Here's how the part is built. I have some questions about the finished solid (model axes, mm). A direction names the side the tool comes from. Give positions to 0.01 mm unless a question says otherwise; leave off trailing zeros. Write each loop counter-clockwise with the first axis right and the second up, starting at its lowest first coordinate (ties: lowest second). Pieces come first, ordered by that corner, then holes. Notation, with made-up numbers: (17.25, 49) - (76.25, 49) arc R16 cw to (76.25, 57) - close; hole circle Ø5 at (28, 18). An arc over 180 degrees is marked (long way). Write each question's results on one line, items separated by ' | '. Start each with the question number.
Item 1: We'd pull the mould along X, two halves only. Please class faces 6 (the cylindrical face through (-23.43, 4.93, 83.45)), 7 (the cylindrical face through (0.22, 6.084, -30.907)), 8 (the cylindrical face through (-65.4, 12.5, 43.2)): +X half, -X half, draft (parallel to the pull), parting line (faces both ways), or undercut.
Item 2: Suppose I cut it at C-C on z = 79. List the corners of the cut face in (x, y) for me.
Item 3: Will these pins go through, and if not, where does the flat tip stop? P1, Ø17.5, axis at x = -54, z = -25.5, coming from the -Y side; P2, Ø1.5, axis at x = 12.5, z = -63.5, coming from the -Y side; P3, Ø4, axis at x = 8.5, y = 13, coming from the -Z side.
Item 4: Which directions (+Z, -Z, +X, -X, +Y, -Y) give clear straight access to the entire face, cutting with the end or side of a thin tool? Please do faces 1 (the cylindrical face through (-65.67, 12.54, 16.84)), 2 (the cylindrical face through (1.033, 12.535, 54.773)), 3 (the flat face through (63.557, 12, -26)), 4 (the cylindrical face through (-59.669, 8.986, -12.754)), 5 (the cylindrical face through (46.448, 12.535, -93.326)).
Item 5: Suppose I cut it at A-A on y = 4.5. Count the separate pieces of the cut face and the enclosed holes in it, then the cut area to 3 significant figures.
Item 6: Please list where these lines run through material, in increasing order: line 1 along Z through (x, y) = (0.5, 10.75); line 2 along X through (y, z) = (4.75, -78.5); line 3 along Y through (x, z) = (-11.5, -62).
Item 7: Suppose I cut it at D-D on x = 19. List the corners of the cut face in (y, z) for me.
```python
from build123d import *
from build123d.topology import SkipClean

# Parameters (mm, degrees)
SKETCH1_R           = 7.5
BOSS_EXTRUDE1_DEPTH = 15
SKETCH4_R           = 5
CUT_EXTRUDE2_DEPTH  = 20
SKETCH5_R           = 11
CUT_EXTRUDE3_DEPTH  = 3
SKETCH6_R           = 1.5
CUT_EXTRUDE4_DEPTH  = 133.338393859
SKETCH7_R           = 8
CUT_EXTRUDE5_DEPTH  = 4
FILLET3_R           = 30
FILLET4_R           = 10
SKETCH9_R           = 23.5
CUT_EXTRUDE6_DEPTH  = 5
SKETCH10_R          = 4
CUT_EXTRUDE7_DEPTH  = 133.172048819
SKETCH11_R          = 12
CUT_EXTRUDE8_DEPTH  = 8
FILLET5_R           = 10
SKETCH12_R          = 4
CUT_EXTRUDE9_DEPTH  = 133.035792455
SKETCH14_R          = 24
SKETCH14_R_2        = 15
CUT_EXTRUDE16_DEPTH = 10
FILLET6_R           = 10
FILLET7_START       = 8
FILLET7_DEPTH       = 2


with BuildPart() as part:
    # Sketch1 → Boss-Extrude1 (new body)
    with BuildSketch(Plane(origin=(0, 0, 0), x_dir=(1, 0, 0), z_dir=(0, 1, 0))):
        with BuildLine():
            Line((-47.707272336, 93.074011467), (46.85801727, 93.074011467))
            ThreePointArc((46.85801727, 93.074011467), (67.451414768, 89.11955675), (63.55694563, 68.514731035))
            Line((63.55694563, 68.514731035), (63.55694563, -17.060551097))
            ThreePointArc((63.55694563, -17.060551097), (70.78018401, -29.882416282), (64.134785378, -43.013070362))
            Line((64.134785378, -43.013070362), (43.994737315, -110.750576059))
            Line((43.994737315, -110.750576059), (-44.651292342, -110.750576059))
            Line((-44.651292342, -110.750576059), (-65.275039181, -42.659888117))
            ThreePointArc((-65.275039181, -42.659888117), (-71.439667546, -30.058632987), (-65, -17.595689691))
            Line((-65, -17.595689691), (-65, 69.228067604))
            ThreePointArc((-65, 69.228067604), (-67.7628182, 89.424810491), (-47.707272336, 93.074011467))
        make_face()
        with Locations(Location((-55.828277514, 80.770057168, 0), (0, 0, 270))):
            Circle(SKETCH1_R, mode=Mode.SUBTRACT)
        with Locations(Location((55.171722486, 80.770057168, 0), (0, 0, 270))):
            Circle(SKETCH1_R, mode=Mode.SUBTRACT)
        with Locations(Location((-55.828277514, -30.229942832, 0), (0, 0, 270))):
            Circle(SKETCH1_R, mode=Mode.SUBTRACT)
        with Locations(Location((55.171722486, -30.229942832, 0), (0, 0, 270))):
            Circle(SKETCH1_R, mode=Mode.SUBTRACT)
    extrude(amount=BOSS_EXTRUDE1_DEPTH)

    # Sketch4 → Cut-Extrude2 (cut)
    with BuildSketch(Plane(origin=(0, 15, 0), x_dir=(1, 0, 0), z_dir=(0, 1, 0))):
        with Locations(Location((0, 25.91137957, 0), (0, 0, 270))):
            Circle(SKETCH4_R)
    extrude(amount=-CUT_EXTRUDE2_DEPTH, mode=Mode.SUBTRACT)

    # Sketch5 → Cut-Extrude3 (cut)
    with BuildSketch(Plane(origin=(0, 15, 0), x_dir=(1, 0, 0), z_dir=(0, 1, 0))):
        with Locations(Location((0, 25.91137957, 0), (0, 0, 270))):
            Circle(SKETCH5_R)
    extrude(amount=-CUT_EXTRUDE3_DEPTH, mode=Mode.SUBTRACT)

    # Sketch6 → Cut-Extrude4 (cut, through all)
    with BuildSketch(Plane(origin=(0, 12, 0), x_dir=(1, 0, 0), z_dir=(0, 1, 0))):
        with Locations(Location((-5.656854249, 31.568233819, 0), (0, 0, 270))):
            Circle(SKETCH6_R)
        with Locations(Location((5.656854249, 31.568233819, 0), (0, 0, 270))):
            Circle(SKETCH6_R)
        with Locations(Location((5.656854249, 20.25452532, 0), (0, 0, 270))):
            Circle(SKETCH6_R)
        with Locations(Location((-5.656854249, 20.25452532, 0), (0, 0, 270))):
            Circle(SKETCH6_R)
    extrude(amount=-CUT_EXTRUDE4_DEPTH, mode=Mode.SUBTRACT)

    # Sketch7 → Cut-Extrude5 (cut)
    with BuildSketch(Plane(origin=(0, 15, 0), x_dir=(1, 0, 0), z_dir=(0, 1, 0))):
        with Locations(Location((0, -15.077036946, 0), (0, 0, 270))):
            Circle(SKETCH7_R)
    extrude(amount=-CUT_EXTRUDE5_DEPTH, mode=Mode.SUBTRACT)

    # Fillet3
    fillet3_edges = [part.edges().sort_by_distance(p)[0] for p in [
        (43.994737315, 7.5, 110.750576059),
        (-44.651292342, 7.5, 110.750576059),
    ]]
    fillet(fillet3_edges, radius=FILLET3_R)

    # Fillet4
    fillet4_edges = [part.edges().sort_by_distance(p)[0] for p in [
        (64.134785378, 7.5, 43.013070362),
        (-65.275039181, 7.5, 42.659888117),
    ]]
    fillet(fillet4_edges, radius=FILLET4_R)

    # Sketch9 → Cut-Extrude6 (cut)
    with BuildSketch(Plane(origin=(0, 15, 0), x_dir=(1, 0, 0), z_dir=(0, 1, 0))):
        with Locations(Location((0, -78.250576059, 0), (0, 0, 270))):
            Circle(SKETCH9_R)
    extrude(amount=-CUT_EXTRUDE6_DEPTH, mode=Mode.SUBTRACT)

    # Sketch10 → Cut-Extrude7 (cut, through all)
    with BuildSketch(Plane(origin=(0, 10, 0), x_dir=(1, 0, 0), z_dir=(0, 1, 0))):
        with Locations(Location((0, -78.250576059, 0), (0, 0, 270))):
            Circle(SKETCH10_R)
    extrude(amount=-CUT_EXTRUDE7_DEPTH, mode=Mode.SUBTRACT)

    # Sketch11 → Cut-Extrude8 (cut)
    with BuildSketch(Plane.XZ):
        with Locations((-55, -25.91137957)):
            Circle(SKETCH11_R)
        with Locations((55, -25.91137957)):
            Circle(SKETCH11_R)
    extrude(amount=-CUT_EXTRUDE8_DEPTH, mode=Mode.SUBTRACT)

    # Fillet5
    fillet5_edges = [part.edges().sort_by_distance(p)[0] for p in [
        (63.55694563, 4, -17.498372885),
        (63.55694563, 4, -34.324386255),
        (-65, 4, -32.544629151),
        (-65, 4, -19.278129989),
    ]]
    fillet(fillet5_edges, radius=FILLET5_R)

    # Sketch12 → Cut-Extrude9 (cut, through all)
    with BuildSketch(Plane.XZ.offset(-8)):
        with Locations(Location((-55, -25.91137957, 0), (0, 0, 270))):
            Circle(SKETCH12_R)
        with Locations(Location((55, -25.91137957, 0), (0, 0, 270))):
            Circle(SKETCH12_R)
    extrude(amount=-CUT_EXTRUDE9_DEPTH, mode=Mode.SUBTRACT)

    # Sketch14 → Cut-Extrude16 (cut)
    with SkipClean():  # the faces are left unmerged after this step: merging them gives an invalid solid
        with BuildSketch(Plane.XZ):
            with BuildLine():
                Line((63.55694563, -3.958757993), (63.55694563, 17.060551097))
                ThreePointArc((63.55694563, 17.060551097), (39.633853338, 31.752922858), (65.954448155, 41.520543922))
                ThreePointArc((65.954448155, 41.520543922), (64.328969033, 43.536593055), (63.275701742, 45.902446917))
                Line((63.275701742, 45.902446917), (50.37240498, 89.300413753))
                ThreePointArc((50.37240498, 89.300413753), (39.553990203, 104.79735475), (21.616531225, 110.750576059))
                Line((21.616531225, 110.750576059), (-22.391974152, 110.750576059))
                ThreePointArc((-22.391974152, 110.750576059), (-40.268031225, 104.843035119), (-51.103852363, 89.447014961))
                Line((-51.103852363, 89.447014961), (-64.46051315, 45.349100617))
                ThreePointArc((-64.46051315, 45.349100617), (-65.439681201, 43.13060481), (-66.9240694, 41.213032024))
                ThreePointArc((-66.9240694, 41.213032024), (-40.267501523, 31.497655875), (-65, 17.595689691))
                Line((-65, 17.595689691), (-65, -3.91137957))
                ThreePointArc((-65, -3.91137957), (-62.071067812, -10.982447382), (-55, -13.91137957))
                ThreePointArc((-55, -13.91137957), (-43, -25.91137957), (-55, -37.91137957))
                ThreePointArc((-55, -37.91137957), (-62.071067812, -40.840311758), (-65, -47.91137957))
                Line((-65, -47.91137957), (-65, -69.228067604))
                ThreePointArc((-65, -69.228067604), (-43.893736828, -72.115303846), (-47.707272336, -93.074011467))
                Line((-47.707272336, -93.074011467), (46.85801727, -93.074011467))
                ThreePointArc((46.85801727, -93.074011467), (42.892030205, -72.420557586), (63.55694563, -68.514731035))
                Line((63.55694563, -68.514731035), (63.55694563, -47.864001147))
                ThreePointArc((63.55694563, -47.864001147), (60.856237995, -41.028773939), (54.212879435, -37.885536794))
                ThreePointArc((54.212879435, -37.885536794), (43, -25.91137957), (54.212879435, -13.937222346))
                ThreePointArc((54.212879435, -13.937222346), (60.856237995, -10.793985201), (63.55694563, -3.958757993))
            make_face()
            with Locations(Location((0, 78.250576059, 0), (0, 0, 270))):
                Circle(SKETCH14_R, mode=Mode.SUBTRACT)
            with Locations(Location((0, -25.91137957, 0), (0, 0, 270))):
                Circle(SKETCH14_R_2, mode=Mode.SUBTRACT)
        extrude(amount=-CUT_EXTRUDE16_DEPTH, mode=Mode.SUBTRACT)

    # Fillet6
    fillet6_edges = [part.edges().sort_by_distance(p)[0] for p in [
        (-47.707272336, 12.5, -93.074011467),
        (46.85801727, 12.5, -93.074011467),
        (63.55694563, 12.5, -68.514731035),
        (63.55694563, 12.5, 17.060551097),
        (-65, 12.5, 17.595689691),
        (-65, 12.5, -69.228067604),
    ]]
    fillet(fillet6_edges, radius=FILLET6_R)

    # Fillet7: read off the stored shape, not the designer's step
    # Fillet7 outline → Fillet7 (cut)
    with SkipClean():  # the faces are left unmerged after this step: merging them gives an invalid solid
        with BuildSketch(Plane(origin=(0, 0, 0), x_dir=(1, 0, 0), z_dir=(0, 1, 0)).offset(FILLET7_START)):
            with BuildLine():
                ThreePointArc((-65, 3.91137957), (-64.534625893, 6.926493016), (-63.181818182, 9.660975316))
                ThreePointArc((-63.181818182, 9.660975316), (-64.301511345, 9.282472301), (-65, 10.23593489))
                Line((-65, 10.23593489), (-65, 3.91137957))
            make_face()
            with BuildLine():
                Line((-65, 47.91137957), (-65, 41.58682425))
                ThreePointArc((-65, 41.58682425), (-64.301511345, 42.540286839), (-63.181818182, 42.161783824))
                ThreePointArc((-63.181818182, 42.161783824), (-64.534625893, 44.896266124), (-65, 47.91137957))
            make_face()
            with BuildLine():
                ThreePointArc((63.55694563, 47.864001147), (63.091571523, 44.848887701), (61.738763812, 42.114405401))
                ThreePointArc((61.738763812, 42.114405401), (62.858456975, 42.492908415), (63.55694563, 41.539445826))
                Line((63.55694563, 41.539445826), (63.55694563, 47.864001147))
            make_face()
            with BuildLine():
                Line((63.55694563, 3.958757993), (63.55694563, 10.283313314))
                ThreePointArc((63.55694563, 10.283313314), (62.858456975, 9.329850724), (61.738763812, 9.708353739))
                ThreePointArc((61.738763812, 9.708353739), (63.091571523, 6.973871439), (63.55694563, 3.958757993))
            make_face()
        extrude(amount=FILLET7_DEPTH, mode=Mode.SUBTRACT)


solid = part.part
```
Checked values:
1) face 6: parting line | face 7: undercut | face 8: -X half
2) outline: (-54.27, 10) - (-23.99, 10) - (-23.99, 0) - (-3.93, 0) - (-3.93, 10) - (-23.49, 10) - (-23.49, 15) - (-54.27, 15) - close; (3.93, 0) - (23.99, 0) - (23.99, 10) - (53.43, 10) - (53.43, 15) - (23.49, 15) - (23.49, 10) - (3.93, 10) - close
3) P1: stops at y = 8 | P2: stops at y = 10 | P3: stops at z = -93.07
4) face 1: -X, +Y, -Y | face 2: +Y | face 3: +X, +Y, -Y | face 4: -Y | face 5: -Z, +Y, -Y
5) separate pieces: 6 | enclosed holes: 10 | area: 4,560 mm^2
6) line 1: z = -93.07 to -30.89, -20.94 to 54.76, 101.75 to 110.75 | line 2: x = -70.39 to -62.98, -48.68 to -41.26, 40.5 to 48.02, 62.32 to 69.85 | line 3: y = 10 to 15
7) outline: (0, 63.59) - (10, 63.59) - (10, -93.07) - (15, -93.07) - (15, 64.42) - (10, 64.42) - (10, 92.08) - (15, 92.08) - (15, 110.75) - (10, 110.75) - (10, 92.91) - (0, 92.91) - close
